Autodesk Inventor part; units mm, degrees
ref_plane "YZ Plane" through (0, 0, 0) normal (1, 0, 0) x (0, 1, 0)
ref_plane "XZ Plane" through (0, 0, 0) normal (0, 1, 0) x (-1, 0, 0)
ref_plane "XY Plane" through (0, 0, 0) normal (0, 0, 1) x (1, 0, 0)
sketch "Sketch1" plane through (0, 0, 0) normal (1, 0, 0) x (0, 1, 0)
  line L0 (0, 0) -> (42, 0)
  line L1 (42, 0) -> (42, 42)
  line L2 (42, 42) -> (0, 42)
  line L3 (0, 42) -> (0, 0)
  dimension "d0" = 42
  dimension "d1" = 42
extrude "Extrusion1" add sketch "Sketch1" against normal blind 37.25
sketch "Sketch2" plane through (0, 0, 0) normal (1, 0, 0) x (0, 0, -1)
  line L0 (-42, 42) -> (0, 42) construction
  line L1 (-21, 42) -> (-21, 0) construction
  line L2 (0, 0) -> (-42, 0) construction
  circle A0 centre (-21, 21) radius 11
  circle A1 centre (-21, 21) radius 4
  dimension "d4" = 22
  dimension "d5" = 8
extrude "Extrusion2" add sketch "Sketch2" along normal blind 2
sketch "Sketch3" plane through (0, 21, 21) normal (1, 0, 0) x (0, 0, -1)
  circle A0 centre (0, 0) radius 4
  circle A1 centre (0, 0) radius 2.5
  point P0 (21, -21)
  dimension "d8" = 5
extrude "Extrusion3" add sketch "Sketch3" along normal blind 22 contours A1
chamfer "Chamfer1" distance 5 angle 45 4 edges at (-18.625, 42, 42) (-18.625, 42, 0) (-18.625, 0, 42) (-18.625, 0, 0)
sketch "Sketch4" plane through (0, 0, 0) normal (1, 0, 0) x (0, 0, -1)
  line L0 (-35.375, 35.3745) -> (-6.625, 35.3745) construction
  line L1 (-6.625, 35.3745) -> (-6.625, 6.6245) construction
  line L2 (-6.625, 6.6245) -> (-35.375, 6.6245) construction
  line L3 (-35.375, 6.6245) -> (-35.375, 35.3745) construction
  line L4 (-42, 37) -> (-42, 5) construction
  line L5 (-5, 42) -> (-37, 42) construction
  circle A0 centre (-6.625, 35.3745) radius 1.25
  circle A1 centre (-35.375, 35.3745) radius 1.25
  circle A2 centre (-35.375, 6.6245) radius 1.25
  circle A3 centre (-6.625, 6.6245) radius 1.25
  point P0 (0, 0)
  dimension "d14" = 28.75
  dimension "d15" = 28.75
  dimension "d16" = 6.625
  dimension "d17" = 6.6255
  dimension "d18" = 2.5
  dimension "d19" = 2.5
  dimension "d20" = 2.5
  dimension "d21" = 2.5
extrude "Extrusion4" cut sketch "Sketch4" against normal blind 5
sketch "Sketch8" plane through (0, 42, 37) normal (0, 1, 0) x (1, 0, 0)
  line L0 (-37.25, 0) -> (-37.25, 32) construction
  line L1 (-37.25, 16) -> (0, 16) construction
  line L2 (0, 18.5) -> (0, 13.5) construction
  line L3 (-37.25, 7.75) -> (-27.25, 7.75)
  line L4 (-27.25, 7.75) -> (-27.25, 24.25)
  line L5 (-27.25, 24.25) -> (-37.25, 24.25)
  line L6 (-37.25, 24.25) -> (-37.25, 7.75)
  point P0 (0, 37)
  dimension "d44" = 10
  dimension "d45" = 16.5
  dimension "d46" = 8.25
extrude "Extrusion8" add sketch "Sketch8" along normal blind 5
equation "\"d46\" = 0.5 * d45"
properties part number "Nema 17 Stepper Motor"
Here's how the part is built. I have some questions about the finished solid (model axes, mm). A direction names the side the tool comes from. Coordinates: 2 decimals unless noted, no trailing zeros. Write each loop counter-clockwise with the first axis right and the second up, starting at its lowest first coordinate (ties: lowest second). Pieces come first, ordered by that corner, then holes.
Item 1: I want a section at A-A on x = -32.5. Write out the boundary of the cut face in (y, z).
Item 2: I want a section at B-B on y = 21. Write out the boundary of the cut face in (x, z).
Item 3: If we mould it in two halves opening along Y, with no side actions, what happens to faces 1 (the flat face through (2, 16, 21)), 2 (the flat face through (-32, 47, 21)), 3 (the flat face through (-5, 35, 35))? For each: +Y half, -Y half, draft (parallel to the pull), parting line (faces both ways), or undercut.
Item 4: I want a section at D-D on x = -10. Write out the boundary of the cut face in (y, z).
Item 5: I want a section at C-C on z = 21. Write out the boundary of the cut face in (x, y).
Item 6: Will these pins go through, and if not, where does the flat tip stop? pin 1 (4 mm diameter, centred on y = 33, z = 14.5, fed in from +X); pin 2 (1.5 mm diameter, centred on y = 35.37, z = 6.62, fed in from +X); pin 3 (1.5 mm diameter, centred on x = -32, y = 45.5, fed in from +Z).
Item 7: If I drill on line 1 (Y direction, x = -2, z = 6); line 2 (X direction, y = 35, z = 10); line 3 (X direction, y = 7.5, z = 35), over which ranges is the centre line in solid material (lowest first)?
Item 8: On a 3-axis mill with a long thin cutter (end or side, diameter ignored), from which of +Z, -Z, +X, -X, +Y, -Y can I reach the whole of each face in a straight line? I mean faces 4 (the flat face through (-37.25, 23, 21)), 5 (the flat face through (-32, 44, 29.25)), 6 (the cylindrical face through (0.99, 18.3, 23.95)), 7 (the flat face through (-27.25, 44, 21)), 8 (the flat face through (-18, 21, 42)). Say none if no direction works.
Findings below:
1. outline: (0, 5) - (5, 0) - (37, 0) - (42, 5) - (42, 12.75) - (47, 12.75) - (47, 29.25) - (42, 29.25) - (42, 37) - (37, 42) - (5, 42) - (0, 37) - close
2. outline: (-37.25, 0) - (0, 0) - (0, 10) - (2, 10) - (2, 17) - (0, 17) - (0, 18.5) - (22, 18.5) - (22, 23.5) - (0, 23.5) - (0, 25) - (2, 25) - (2, 32) - (0, 32) - (0, 42) - (-37.25, 42) - close
3. face 1: draft
3. face 2: +Y half
3. face 3: undercut
4. outline: (0, 5) - (5, 0) - (37, 0) - (42, 5) - (42, 37) - (37, 42) - (5, 42) - (0, 37) - close
5. outline: (-37.25, 0) - (0, 0) - (0, 10) - (2, 10) - (2, 17) - (0, 17) - (0, 18.5) - (22, 18.5) - (22, 23.5) - (0, 23.5) - (0, 25) - (2, 25) - (2, 32) - (0, 32) - (0, 42) - (-27.25, 42) - (-27.25, 47) - (-37.25, 47) - close
6. pin 1: stops at x = 0
6. pin 2: stops at x = -5
6. pin 3: stops at z = 29.25
7. line 1: y = 0 to 5.54, 7.71 to 34.29, 36.46 to 42
7. line 2: x = -37.25 to 0
7. line 3: x = -37.25 to -5
8. face 4: +Z, -Z, -X, +Y, -Y
8. face 5: +Z, +X, -X, +Y
8. face 6: +X
8. face 7: +Z, -Z, +X, +Y
8. face 8: +Z, +X, -X, +Y, -Y
